Geometry: final body of the model. Coordinates: model frame, mm. A direction names the side the tool comes from. Round coordinates to 2 decimals unless told otherwise and drop trailing zeros. Loops run counter-clockwise (first coordinate to the right, second up) from the corner with the lowest first, then second, coordinate; pieces in that order, holes last. Notation, with made-up numbers: (53, 83.5) - (80, 83.5) arc R31 cw to (80, 116.5) - close; hole circle Ø3 at (3.25, 39.5). An arc over 180 degrees is marked (long way). Answer in a Markdown table with one row per item. Add a question column.
from build123d import *

# Parameters (mm, degrees)
SKETCH1_W           = 90
SKETCH1_H           = 125
BOSS_EXTRUDE1_DEPTH = 4
SKETCH2_W           = 90
SKETCH2_H           = 125
SKETCH2_W_2         = 86
SKETCH2_H_2         = 121
BOSS_EXTRUDE2_DEPTH = 2
SKETCH3_W           = 20.5
SKETCH3_H           = 12
CUT_EXTRUDE1_DEPTH  = 10


with BuildPart() as part:
    # Sketch1 → Boss-Extrude1 (new body)
    with BuildSketch(Plane(origin=(0, 55.343226389, 0), x_dir=(1, 0, 0), z_dir=(0, 1, 0))):
        Polygon((-104.681843773, -215.861584775), (-104.681843773, -229.045240407), (-59.681843773, -229.045240407), (-59.681843773, -215.861584775), (32.818156227, -215.861584775), (32.818156227, -70.861584775), (-137.181843773, -70.861584775), (-137.181843773, -215.861584775), align=None)
        with Locations((-82.181843773, -143.361584775)):
            Rectangle(SKETCH1_W, SKETCH1_H, mode=Mode.SUBTRACT)
    extrude(amount=BOSS_EXTRUDE1_DEPTH)

    # Sketch2 → Boss-Extrude2 (add)
    with BuildSketch(Plane(origin=(0, 59.343226389, 0), x_dir=(1, 0, 0), z_dir=(0, 1, 0))):
        with Locations((-82.181843773, -143.361584775)):
            Rectangle(SKETCH2_W, SKETCH2_H)
        with Locations((-82.181843773, -143.361584775)):
            Rectangle(SKETCH2_W_2, SKETCH2_H_2, mode=Mode.SUBTRACT)
    extrude(amount=-BOSS_EXTRUDE2_DEPTH)

    # Sketch3 → Cut-Extrude1 (cut)
    with BuildSketch(Plane(origin=(0, 59.343226389, 0), x_dir=(1, 0, 0), z_dir=(0, 1, 0))):
        with Locations((-49.431843773, -209.861584775)):
            Rectangle(SKETCH3_W, SKETCH3_H)
    extrude(amount=-CUT_EXTRUDE1_DEPTH, mode=Mode.SUBTRACT)


solid = part.part
1) Section B-B, the plane x = -81. Return the cut outline in (y, z).
2) Section C-C, the plane z = 89. Return the cut outline in (x, y), and give its area (3 significant figures).
3) Pull-direction query (Z, two-part tool) for faces 1 (the flat face through (-126, 57.343, 143)), 2 (the flat face through (-51, 57, 70.862)), 3 (the flat face through (-4, 57, 215.862)), 4 (the flat face through (-34, 55.343, 131)); classes: pulls with the +Z half, pulls with the -Z half, needs draft (parallel to the pull), parting line crosses it, or undercut.
4) Reachability of faces 5 (the flat face through (-121, 57, 215.862)), 6 (the flat face through (32.818, 57, 144)), 7 (the flat face through (-39.182, 58, 150)) from +Z, -Z, +X, -X, +Y, -Y: full face, straight path, thin tool, end or side. Return the list, or none.
5) Section D-D, the plane y = 58.7. Return the cut outline in (x, z), and give its area (3 significant figures).
6) Material intervals for line 1 along X through (y, z) = (57.15, 189); line 2 along X through (y, z) = (58.65, 174); line 3 along Z through (x, y) = (-96, 57.8), sorted ascending. Write a range as from..to.
7) Contact query for a flat-ended pin moving along its axis: pin 1 Ø2 at (x, y) = (-2.5, 56.5) entering from +Z. Output: stop coordinate, or through.
8) Section A-A, the plane z = 212.5. Return the cut outline in (x, y).
Evaluation:
| question | item | result |
|---|---|---|
| 1 | outline | (55.34, 70.86) - (59.34, 70.86) - (59.34, 82.86) - (57.34, 82.86) - (57.34, 80.86) - (55.34, 80.86) - close; (55.34, 205.86) - (57.34, 205.86) - (57.34, 203.86) - (59.34, 203.86) - (59.34, 229.05) - (55.34, 229.05) - close |
| 2 | outline | (-137.18, 55.34) - (-127.18, 55.34) - (-127.18, 57.34) - (-125.18, 57.34) - (-125.18, 59.34) - (-137.18, 59.34) - close; (-39.18, 57.34) - (-37.18, 57.34) - (-37.18, 55.34) - (32.82, 55.34) - (32.82, 59.34) - (-39.18, 59.34) - close |
| 2 | area | 328 mm² |
| 3 | face 1 | undercut |
| 3 | face 2 | pulls with the -Z half |
| 3 | face 3 | pulls with the +Z half |
| 3 | face 4 | needs draft |
| 4 | face 5 | +Z, -X, +Y, -Y |
| 4 | face 6 | +Z, -Z, +X, +Y, -Y |
| 4 | face 7 | +Z, +Y, -Y |
| 5 | outline | (-137.18, 70.86) - (32.82, 70.86) - (32.82, 215.86) - (-39.18, 215.86) - (-39.18, 82.86) - (-125.18, 82.86) - (-125.18, 203.86) - (-59.68, 203.86) - (-59.68, 229.05) - (-104.68, 229.05) - (-104.68, 215.86) - (-137.18, 215.86) - close |
| 5 | area | 14,600 mm² |
| 6 | line 1 | x = -137.18..-127.18, -37.18..32.82 |
| 6 | line 2 | x = -137.18..-125.18, -39.18..32.82 |
| 6 | line 3 | z = 70.86..82.86, 203.86..229.05 |
| 7 | pin 1 | stops at z = 215.86 |
| 8 | outline | (-137.18, 55.34) - (-59.68, 55.34) - (-59.68, 59.34) - (-137.18, 59.34) - close; (-39.18, 55.34) - (32.82, 55.34) - (32.82, 59.34) - (-39.18, 59.34) - close |
